```python
from build123d import *

# Parameters (mm, degrees)
SKETCH_W        = 17.15
SKETCH_H        = 37
PAD_DEPTH       = 11
SKETCH001_W     = 12.6
SKETCH001_H     = 32.7
POCKET_DEPTH    = 2.7
SKETCH002_W     = 12.6
SKETCH002_H     = 23
POCKET001_DEPTH = 4
POCKET002_DEPTH = 4.3
SKETCH004_R     = 1.2
POCKET003_DEPTH = 8.301


with BuildPart() as part:
    # Sketch → Pad (new body)
    with BuildSketch(Plane.XY):
        with Locations((8.575, 18.5)):
            Rectangle(SKETCH_W, SKETCH_H)
    extrude(amount=PAD_DEPTH)

    # Sketch001 (on Face6 of Pad) → Pocket (cut)
    with BuildSketch(Plane.XY.offset(11)):
        with Locations((8.575, 18.5)):
            Rectangle(SKETCH001_W, SKETCH001_H)
    extrude(amount=-POCKET_DEPTH, mode=Mode.SUBTRACT)

    # Sketch002 (on Face11 of Pocket) → Pocket001 (cut)
    with BuildSketch(Plane.XY.offset(8.3)):
        with Locations((8.575, 18.5)):
            Rectangle(SKETCH002_W, SKETCH002_H)
    extrude(amount=-POCKET001_DEPTH, mode=Mode.SUBTRACT)

    # Sketch003 (on Face17 of Pocket001) → Pocket002 (cut)
    with BuildSketch(Plane.XY.offset(4.3)):
        with BuildLine():
            ThreePointArc((11.725, 18.24404), (8.575, 30), (5.425, 18.24404))
            ThreePointArc((5.425, 18.24404), (8.575, 15.09404), (11.725, 18.24404))
        make_face()
    extrude(amount=-POCKET002_DEPTH, mode=Mode.SUBTRACT)

    # Sketch004 (on Face18 of Pocket002) → Pocket003 (cut, through all)
    with BuildSketch(Plane.XY.offset(8.3)):
        with Locations((8.575, 32.15)):
            Circle(SKETCH004_R)
        with Locations((8.575, 4.85)):
            Circle(SKETCH004_R)
    extrude(amount=-POCKET003_DEPTH, mode=Mode.SUBTRACT)


solid = part.part
```
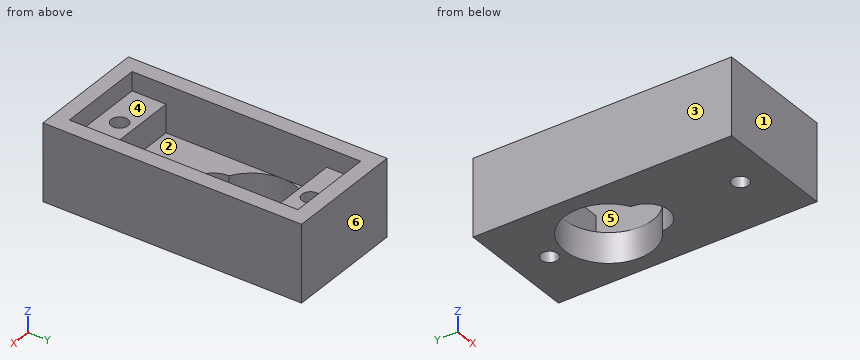
Verification items for the finished model (mm, model axes). Face numbers are marked on the shaded views. A direction names the side the tool comes from. Give positions to 0.01 mm unless a question says otherwise; leave off trailing zeros. Write each loop counter-clockwise with the first axis right and the second up, starting at its lowest first coordinate (ties: lowest second). Pieces come first, ordered by that corner, then holes. Notation, with made-up numbers: M 67.5,-28.5 L 121.5,-28.5 A23 ccw 121.5,-1.5 Z; hole C 55.25,-8.5 d11. An arc over 180 degrees is marked long. One line per question, with ' | ' between items.
1) Thickness scan on line 1 along Y through (x, z) = (10, 8); line 2 along Y through (x, z) = (8.5, 1.75); line 3 along X through (y, z) = (13, 5.5) (3 decimals). Record the ranges inside material, lowest first. Write a range as [from, to].
Result:
line 1: y = [0, 7], [30, 37] | line 2: y = [0, 3.65], [6.05, 15.09], [30, 30.95], [33.35, 37] | line 3: x = [0, 2.275], [14.875, 17.15]
2) Gauge pin test, flat ends, axial feed: pin 1 Ø4 at (x, y) = (8.575, 32.15) entering from +Z; pin 2 Ø7 at (x, y) = (6, 26) entering from +Z. Record the tip position at first contact, or that the pin passes through.
Result:
pin 1: stops at z = 8.3 | pin 2: stops at z = 4.3
3) Section check B-B on y = 32.15. Enter the section's corners in (x, z) (3 decimals), plus the area to 3 significant figures.
Result:
outline: M 0,0 L 7.375,0 L 7.375,8.3 L 2.275,8.3 L 2.275,11 L 0,11 Z; M 9.775,0 L 17.15,0 L 17.15,11 L 14.875,11 L 14.875,8.3 L 9.775,8.3 Z | area: 135 mm2
4) Section check C-C on x = 12.5. Enter the section's corners in (y, z).
Result:
outline: M 0,0 L 18.77,0 L 18.77,4.3 L 7,4.3 L 7,8.3 L 2.15,8.3 L 2.15,11 L 0,11 Z; M 28.63,0 L 37,0 L 37,11 L 34.85,11 L 34.85,8.3 L 30,8.3 L 30,4.3 L 28.63,4.3 Z
5) Section check D-D on z = 10. Enter the section's corners in (x, y) (3 decimals).
Result:
outline: M 0,0 L 17.15,0 L 17.15,37 L 0,37 Z; hole M 2.275,2.15 L 14.875,2.15 L 14.875,34.85 L 2.275,34.85 Z
6) Mould release check, pull along X, two halves, no side actions. Record for the marked faces 3, 4, 5 and 6: released by +X, released by -X, zero draft, split by the parting line, or undercut.
Result:
face 3: released by -X | face 4: undercut | face 5: undercut | face 6: zero draft
7) Section check A-A on z = 3. Enter the section's corners in (x, y) (3 decimals), plus the area to 3 significant figures.
Result:
outline: M 0,0 L 17.15,0 L 17.15,37 L 0,37 Z; hole M 5.425,18.244 A3.15 ccw 11.725,18.244 A6.3 ccw long Z; hole C 8.575,4.85 d2.4; hole C 8.575,32.15 d2.4 | area: 489 mm2
8) Set-up check for the marked faces 1 and 2: record each of +Z, -Z, +X, -X, +Y, -Y from which the full face is reachable in a straight line by a thin tool's end or side.
Result:
face 1: +Z, -Z, +X, -X, -Y | face 2: +Z
